Geometry: final body of the model. Coordinates: model frame, mm. Face numbers are marked on the shaded views. A direction names the side the tool comes from. Round coordinates to 2 decimals unless told otherwise and drop trailing zeros. Write each loop counter-clockwise with the first axis right and the second up, starting at its lowest first coordinate (ties: lowest second). Pieces come first, ordered by that corner, then holes. Notation, with made-up numbers: M -27.5,51 L 6.5,51 A29 ccw 6.5,75 Z; hole C 61,-13 d11. An arc over 180 degrees is marked long. Use one line per item in the form item = value. Start each with the question number.
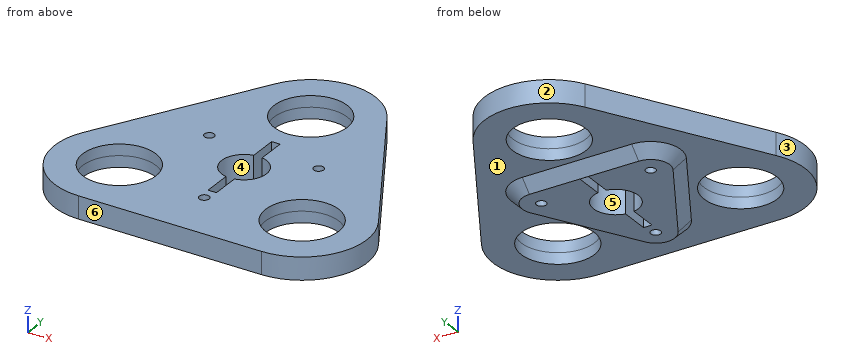
from build123d import *
from build123d.topology import SkipClean

# Parameters (mm, degrees)
SKETCH1_R           = 23.025
SKETCH1_R_2         = 13.025
SKETCH1_R_3         = 7.975
BOSS_EXTRUDE1_DEPTH = 4
BOSS_EXTRUDE3_START = 4
SKETCH5_R           = 7.975
BOSS_EXTRUDE3_DEPTH = 4
CHAMFER2_SIZE       = 4
CUT_EXTRUDE1_DEPTH  = 84.155314152
SKETCH3_R           = 1.75
CUT_EXTRUDE2_DEPTH  = 84.155314152
CIRPATTERN2_COUNT   = 3
CIRPATTERN3_COUNT   = 2


with BuildPart() as part:
    # Sketch1 → Boss-Extrude1 (new, symmetric)
    # profile 1 of 4: a face of its own
    with BuildSketch(Plane.XY):
        with Locations((0, 37.625)):
            Circle(SKETCH1_R)
        with Locations((0, 37.625)):
            Circle(SKETCH1_R_2, mode=Mode.SUBTRACT)
    # profile 2 of 4: a face of its own
    with BuildSketch(Plane.XY):
        with BuildLine():
            ThreePointArc((23.025, 37.625), (-5.959308513, 15.38455785), (-19.940234922, 49.1375))
            Line((-19.940234922, 49.1375), (-52.52444074, -7.3))
            ThreePointArc((-52.52444074, -7.3), (-26.624897304, 3.42794215), (-9.559205817, -18.8125))
            ThreePointArc((-9.559205817, -18.8125), (-16.303072181, -35.093633637), (-32.584205817, -41.8375))
            Line((-32.584205817, -41.8375), (32.584205817, -41.8375))
            ThreePointArc((32.584205817, -41.8375), (12.643970895, -7.3), (52.52444074, -7.3))
            Line((52.52444074, -7.3), (19.940234922, 49.1375))
            ThreePointArc((19.940234922, 49.1375), (22.24044215, 43.584308513), (23.025, 37.625))
        make_face()
        Circle(SKETCH1_R_3, mode=Mode.SUBTRACT)
    # profile 3 of 4: a face of its own
    with BuildSketch(Plane.XY):
        with Locations((-32.584205817, -18.8125)):
            Circle(SKETCH1_R)
        with Locations((-32.584205817, -18.8125)):
            Circle(SKETCH1_R_2, mode=Mode.SUBTRACT)
    # profile 4 of 4: a face of its own
    with BuildSketch(Plane.XY):
        with Locations((32.584205817, -18.8125)):
            Circle(SKETCH1_R)
        with Locations((32.584205817, -18.8125)):
            Circle(SKETCH1_R_2, mode=Mode.SUBTRACT)
    extrude(amount=BOSS_EXTRUDE1_DEPTH, both=True)

    # Sketch5 → Boss-Extrude3 (add)
    with SkipClean():  # the faces are left unmerged after this step: merging them gives an invalid solid
        with BuildSketch(Plane(origin=(0, 0, -4), x_dir=(-1, 0, 0), z_dir=(0, 0, -1)).offset(BOSS_EXTRUDE3_START)):
            with BuildLine():
                Line((-5.845671476, -25.875), (-25.331243061, 7.875))
                ThreePointArc((-25.331243061, 7.875), (-25.331243061, 14.625), (-19.485571585, 18))
                Line((-19.485571585, 18), (19.485571585, 18))
                ThreePointArc((19.485571585, 18), (25.331243061, 14.625), (25.331243061, 7.875))
                Line((25.331243061, 7.875), (5.845671476, -25.875))
                ThreePointArc((5.845671476, -25.875), (0, -29.25), (-5.845671476, -25.875))
            make_face()
            Circle(SKETCH5_R, mode=Mode.SUBTRACT)
        extrude(amount=-BOSS_EXTRUDE3_DEPTH)

    # Chamfer2
    chamfer2_edges = [part.edges().sort_by_distance(p)[0] for p in [
        (0, -29.25, -4),
        (-15.588457268, -9, -4),
        (15.588457268, -9, -4),
        (-25.331243061, 14.625, -4),
        (25.331243061, 14.625, -4),
        (0, 18, -4),
    ]]
    chamfer(chamfer2_edges, length=CHAMFER2_SIZE - 0.0001)  # a hair under: the kernel refuses the full size

    # Sketch2 → Cut-Extrude1 (cut, through all)
    with BuildSketch(Plane.XY.offset(4)):
        with BuildLine():
            Line((-1.5, 17.975), (-1.5, 7.832663978))
            ThreePointArc((-1.5, 7.832663978), (0, 7.975), (1.5, 7.832663978))
            Line((1.5, 7.832663978), (1.5, 17.975))
            Line((1.5, 17.975), (-1.5, 17.975))
        make_face()
    cut_extrude1 = extrude(amount=-CUT_EXTRUDE1_DEPTH, mode=Mode.SUBTRACT)

    # Sketch3 → Cut-Extrude2 (cut, through all)
    with BuildSketch(Plane.XY.offset(4)):
        with Locations((-19.485571585, 11.25)):
            Circle(SKETCH3_R)
    cut_extrude2 = extrude(amount=-CUT_EXTRUDE2_DEPTH, mode=Mode.SUBTRACT)

    # CirPattern2: Cut-Extrude2 ×3 about axis
    cirpattern2_axis = Axis((0, 0, 0), (0, 0, 1))
    for i in range(1, CIRPATTERN2_COUNT):
        add(cut_extrude2.rotate(cirpattern2_axis, i * 360 / CIRPATTERN2_COUNT), mode=Mode.SUBTRACT)

    # CirPattern3: Cut-Extrude1 ×2 about axis
    cirpattern3_axis = Axis((0, 0, 0), (0, 0, 1))
    for i in range(1, CIRPATTERN3_COUNT):
        add(cut_extrude1.rotate(cirpattern3_axis, i * 360 / CIRPATTERN3_COUNT), mode=Mode.SUBTRACT)


solid = part.part
1. Section query B-B (x = 42). Return loops of the section in (y, z), then the cut area to 3 significant figures.
2. Set-up query: the marked faces 5 and 6. Return all of +Z, -Z, +X, -X, +Y, -Y with unobstructed straight access to the full face (end or side cutting, diameter ignored); none if empty.
3. Ray query, probe 1 along Y at (x, z) = (-4, 2); probe 2 along Y at (x, z) = (-7, -3.5); probe 3 along X at (y, z) = (12.5, 3). Return the intervals inside material, ascending.
4. Contact query for flat-ended pins moving along their axis: pin 1 (1 mm diameter, centred on x = 37.5, y = 8, fed in from -Z); pin 2 (21 mm diameter, centred on x = -32.58, y = -18.81, fed in from -Z); pin 3 (1.5 mm diameter, centred on y = -12, z = -2.5, fed in from -X); pin 4 (5 mm diameter, centred on x = 37, z = -4.5, fed in from -Y). Output: stop coordinate, or through.
5. Pull-direction query (X, two-part tool) for the marked faces 1, 2, 3 and 4; classes: released by +X, released by -X, zero draft, split by the parting line, or undercut.
6. Section query C-C (y = 11.25). Give the number of separate pieces and of enclosed holes in the cut face, then the cut area to 3 significant figures.
7. Section query A-A (y = 47). Return loops of the section in (x, z), then the cut area to 3 significant figures.
Checks:
q1.outline = M -39.82,-4 L -27.81,-4 L -27.81,4 L -39.82,4 Z; M -9.81,-4 L 10.93,-4 L 10.93,4 L -9.81,4 Z
q1.area = 262 mm^2
q2.face_5 = +Z, -Z
q2.face_6 = +Z, -Z, +X, -X, -Y
q3.probe_1 = -41.84 to -6.9, 6.9 to 25.23, 50.02 to 60.3
q3.probe_2 = -41.84 to -3.82, 3.82 to 26.64, 48.61 to 59.56
q3.probe_3 = -41.09 to -20.71, -18.26 to -1.5, 1.5 to 18.26, 20.71 to 41.09
q4.pin_1 = -4
q4.pin_2 = through
q4.pin_3 = -54.8
q4.pin_4 = -41.75
q5.face_1 = zero draft
q5.face_2 = split by the parting line
q5.face_3 = released by -X
q5.face_4 = undercut
q6.separate_pieces = 4
q6.enclosed_holes = 0
q6.area = 775 mm^2
q7.outline = M -21.17,-4 L -9.04,-4 L -9.04,4 L -21.17,4 Z; M 9.04,-4 L 21.17,-4 L 21.17,4 L 9.04,4 Z
q7.area = 194 mm^2
